The model under review builds one solid part; all positions refer to its coordinate system, in mm. A direction names the side the tool comes from. Give positions to 0.01 mm unless a question says otherwise; leave off trailing zeros. Loops run counter-clockwise (first coordinate to the right, second up) from the corner with the lowest first, then second, coordinate; pieces in that order, holes last. Notation, with made-up numbers: (7, 85.5) - (55, 85.5) arc R19 cw to (55, 103.5) - close; hole circle Ø2 at (82, 81). An arc over 180 degrees is marked (long way). Answer as a JSON object with one key per item and string values.
from build123d import *

# Parameters (mm, degrees)
SKETCH_3_W          = 13
SKETCH_3_H          = 11
EXTRUDE_1_DEPTH     = 10
SKETCH_5_R          = 2.75
CUT_EXTRUDE_3_DEPTH = 18.298843892
SKETCH_5_6_R        = 0.75
EXTRUDE_2_DEPTH     = 1
SKETCH_10_W         = 7
SKETCH_10_H         = 8
CUT_EXTRUDE_5_DEPTH = 12.947803145
SKETCH_11_W         = 0.5
SKETCH_11_H         = 8
CUT_EXTRUDE_6_DEPTH = 12.947803145


with BuildPart() as part:
    # Sketch 3 → Extrude 1 (new body)
    with BuildSketch(Plane(origin=(0, 0, 0), x_dir=(1, 0, 0), z_dir=(0, 1, 0))):
        Rectangle(SKETCH_3_W, SKETCH_3_H)
    extrude(amount=EXTRUDE_1_DEPTH)

    # Sketch 5 → Cut-Extrude 3 (cut, through all)
    with BuildSketch(Plane(origin=(6.5, 0, 0), x_dir=(0, 0, -1), z_dir=(1, 0, 0))):
        with Locations((-1, 3.5)):
            Circle(SKETCH_5_R)
        with BuildLine():
            Line((-5.5, 10), (-5.5, 2))
            ThreePointArc((-5.5, 2), (-3.889087297, 5.889087297), (0, 7.5))
            Line((0, 7.5), (0.590375146, 6.432854109))
            Line((0.590375146, 6.432854109), (3.698964751, 4.606439417))
            ThreePointArc((3.698964751, 4.606439417), (4.972488989, 4.078928406), (5.5, 2.805404168))
            Line((5.5, 2.805404168), (5.5, 10))
            Line((5.5, 10), (-5.5, 10))
        make_face()
    extrude(amount=-CUT_EXTRUDE_3_DEPTH, mode=Mode.SUBTRACT)

    # Sketch 5_6 → Extrude 2 (add)
    with BuildSketch(Plane(origin=(6.5, 0, 0), x_dir=(0, 0, -1), z_dir=(1, 0, 0))):
        with Locations(Location((4.376425526, 2, 0), (0, 0, 180))):
            Circle(SKETCH_5_6_R)
    extrude_2 = extrude(amount=EXTRUDE_2_DEPTH)

    # Sketch 10 → Cut-Extrude 5 (cut, through all)
    with BuildSketch(Plane.XZ):
        with Locations((0, 1.5)):
            Rectangle(SKETCH_10_W, SKETCH_10_H)
    extrude(amount=-CUT_EXTRUDE_5_DEPTH, mode=Mode.SUBTRACT)

    # Mirror 1: Extrude 2 across plane
    add(extrude_2.mirror(Plane(origin=(0, 0, 0), x_dir=(0, 0, 1), z_dir=(1, 0, 0))))

    # Sketch 11 → Cut-Extrude 6 (cut, through all)
    with BuildSketch(Plane(origin=(0, 0, 0), x_dir=(-1, 0, 0), z_dir=(0, -1, 0))):
        with Locations((-3.75, -1.5)):
            Rectangle(SKETCH_11_W, SKETCH_11_H)
        with Locations((3.75, -1.5)):
            Rectangle(SKETCH_11_W, SKETCH_11_H)
    extrude(amount=-CUT_EXTRUDE_6_DEPTH, mode=Mode.SUBTRACT)


solid = part.part
Q1. Consider section A-A, the plane z = 2. State the section outline as (x, y) points.
Results:
{"outline": "(-6.5, 0) - (-4, 0) - (-4, 0.94) - (-6.5, 0.94) - close; (-6.5, 6.06) - (-4, 6.06) - (-4, 7.12) - (-6.5, 7.12) - close; (4, 0) - (6.5, 0) - (6.5, 0.94) - (4, 0.94) - close; (4, 6.06) - (6.5, 6.06) - (6.5, 7.12) - (4, 7.12) - close"}
Q2. Consider section C-C, the plane y = 5.5. State the section outline as (x, z) points.
Results:
{"outline": "(-6.5, -2.18) - (-4, -2.18) - (-4, -0.89) - (-6.5, -0.89) - close; (-6.5, 2.89) - (-4, 2.89) - (-4, 4.24) - (-6.5, 4.24) - close; (4, -2.18) - (6.5, -2.18) - (6.5, -0.89) - (4, -0.89) - close; (4, 2.89) - (6.5, 2.89) - (6.5, 4.24) - (4, 4.24) - close"}
Q3. Consider section D-D, the plane x = 2.5. State the section outline as (y, z) points.
Results:
{"outline": "(0, -5.5) - (2.81, -5.5) arc R1.8 ccw to (4.61, -3.7) - (5.31, -2.5) - (0, -2.5) - close"}
Q4. To check wall thickness, follow probe 1 along X at (y, z) = (6.5, 2.5); probe 2 along Y at (x, z) = (5.25, 1); probe 3 along Z at (x, y) = (-4.5, 2). State the ranges of each line that lie inside material, in increasing order. Write a range as [from, to].
Results:
{"probe 1": "x = [-6.5, -4], [4, 6.5]", "probe 2": "y = [0, 0.75], [6.25, 7.41]", "probe 3": "z = [-5.5, -1.3], [3.3, 5.5]"}
Q5. Clearance check with flat-ended pins moving along their axes: pin 1 Ø1.6 at (x, y) = (1.5, 2.5) entering from +Z; pin 2 Ø2 at (y, z) = (4, -4) entering from +X; pin 3 Ø1.5 at (y, z) = (2.5, -1) entering from -X. State where each tip first meets the part, or that it passes through.
Results:
{"pin 1": "stops at z = -2.5", "pin 2": "stops at x = 6.5", "pin 3": "stops at x = -6.5"}
Q6. Consider section B-B, the plane y = 3. State the section outline as (x, z) points.
Results:
{"outline": "(-6.5, -5.49) - (6.5, -5.49) - (6.5, -1.7) - (4, -1.7) - (4, -2.5) - (-4, -2.5) - (-4, -1.7) - (-6.5, -1.7) - close; (-6.5, 3.7) - (-4, 3.7) - (-4, 5.41) - (-6.5, 5.41) - close; (4, 3.7) - (6.5, 3.7) - (6.5, 5.41) - (4, 5.41) - close"}
Q7. For faces 1 (the face through (-5.23, 5.85, 3.93)), 2 (the face through (0, 3, -2.5)), 3 (the face through (-6.993, 1.775, -3.661)), list the 3-axis set-ups (+Z, -Z, +X, -X, +Y, -Y) from which the entire face can be reached by the end or side of a thin tool; tool diameter is ignored.
Results:
{"face 1": "+Z, +X, -X, +Y", "face 2": "+Z, +Y, -Y", "face 3": "-X"}
Q8. The part is to be moulded in two halves that separate along Y. For faces 4 (the face through (6.993, 1.775, -3.661)), 5 (the face through (5, 1, 5.5)), 6 (the face through (-5.232, 0.815, 1.596)), say which applies: +Y half, -Y half, draft (parallel to the pull), parting line (faces both ways), or undercut.
Results:
{"face 4": "parting line", "face 5": "draft", "face 6": "undercut"}
